Verification items for the finished model (mm, model axes). Face numbers are marked on the shaded views. A direction names the side the tool comes from. Round coordinates to 2 decimals unless told otherwise and drop trailing zeros. Write each loop counter-clockwise with the first axis right and the second up, starting at its lowest first coordinate (ties: lowest second). Pieces come first, ordered by that corner, then holes. Notation, with made-up numbers: M 86,-36 L 122,-36 A30 cw 122,-8 Z; hole C 7.25,44 d2. An arc over 180 degrees is marked long. Write each question's results on one line, items separated by ' | '.
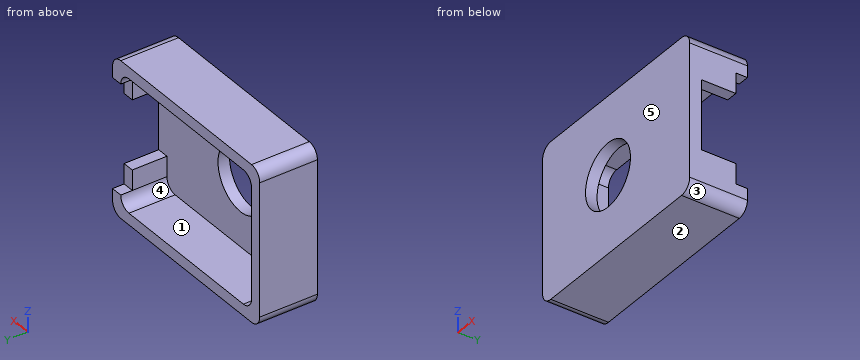
from build123d import *

# Parameters (mm, degrees)
SKETCH1_W           = 36
SKETCH1_H           = 27
SKETCH1_R           = 5.5
BOSS_EXTRUDE1_DEPTH = 2
BOSS_EXTRUDE2_DEPTH = 8
SKETCH3_W           = 3.5
SKETCH3_H           = 6
BOSS_EXTRUDE3_DEPTH = 2
FILLET2_R           = 2


with BuildPart() as part:
    # Sketch1 → Boss-Extrude1 (new body)
    with BuildSketch(Plane(origin=(0, 0, 0), x_dir=(1, 0, 0), z_dir=(0, 1, 0))):
        Rectangle(SKETCH1_W, SKETCH1_H)
        with Locations(Location((-2, 0, 0), (0, 0, 270))):
            Circle(SKETCH1_R, mode=Mode.SUBTRACT)
    extrude(amount=BOSS_EXTRUDE1_DEPTH)

    # Sketch2 → Boss-Extrude2 (add)
    with BuildSketch(Plane(origin=(0, 2, 0), x_dir=(1, 0, 0), z_dir=(0, 1, 0))):
        Polygon((18, 13.5), (-18, 13.5), (-18, -13.5), (18, -13.5), (18, -9.5), (16, -9.5), (16, -11.5), (-16, -11.5), (-16, 11.5), (16, 11.5), (16, 9.5), (18, 9.5), align=None)
    extrude(amount=BOSS_EXTRUDE2_DEPTH)

    # Sketch3 → Boss-Extrude3 (add)
    with BuildSketch(Plane(origin=(18, 0, 0), x_dir=(0, 0, -1), z_dir=(1, 0, 0))):
        with Locations((-7.75, 5)):
            Rectangle(SKETCH3_W, SKETCH3_H)
        with Locations((7.75, 5)):
            Rectangle(SKETCH3_W, SKETCH3_H)
    extrude(amount=-BOSS_EXTRUDE3_DEPTH)

    # Fillet2
    fillet2_edges = [part.edges().sort_by_distance(p)[0] for p in [
        (-18, 5, 13.5),
        (-18, 5, -13.5),
        (18, 5, -13.5),
        (18, 5, 13.5),
        (16, 6, -11.5),
        (16, 6, 11.5),
        (-16, 6, 11.5),
        (-16, 6, -11.5),
    ]]
    fillet(fillet2_edges, radius=FILLET2_R - 0.0001)  # a hair under: the kernel refuses the full size


solid = part.part
1) Sectioned sample at B-B, the plane x = -2. Record the cut outline in (y, z).
Calculated:
outline: M 0,-13.5 L 10,-13.5 L 10,-11.5 L 2,-11.5 L 2,-5.5 L 0,-5.5 Z; M 0,5.5 L 2,5.5 L 2,11.5 L 10,11.5 L 10,13.5 L 0,13.5 Z
2) Draft check along X on the marked faces 1, 2 and 3. Enter one of: pulls with the +X half, pulls with the -X half, needs draft (parallel to the pull), parting line crosses it, or undercut.
Calculated:
face 1: undercut | face 2: needs draft | face 3: pulls with the +X half
3) Sectioned sample at A-A, the plane z = 0. Record the cut outline in (x, y).
Calculated:
outline: M -18,0 L -7.5,0 L -7.5,2 L -16,2 L -16,10 L -18,10 Z; M 3.5,0 L 18,0 L 18,2 L 3.5,2 Z
4) Depth check by flat-ended pin: P1, Ø0.6, axis at x = 16.5, y = 6.5, coming from the -Z side; P2, Ø1, axis at x = 16.5, z = -7.5, coming from the +Y side; P3, Ø3, axis at x = -7.5, z = 9.5, coming from the +Y side. Enter the tip coordinate at first touch or a pass-through.
Calculated:
P1: stops at z = -13.49 | P2: stops at y = 8 | P3: stops at y = 2
5) Sectioned sample at D-D, the plane z = 7. Record the cut outline in (x, y).
Calculated:
outline: M -18,0 L 18,0 L 18,8 L 16,8 L 16,2 L -16,2 L -16,10 L -18,10 Z
6) Access from +Z, -Z, +X, -X, +Y, -Y to the whole of each face (thin tool, end or side, straight path). Record for the marked faces 4 and 5.
Calculated:
face 4: +Y | face 5: +Z, -Z, +X, -X, -Y
7) Material ranges on line 1 (Z direction, x = 6.5, y = 4.25); line 2 (X direction, y = 1.25, z = 0); line 3 (Y direction, x = 0.5, z = 6.25), recorded low to high. Write a range as [from, to].
Calculated:
line 1: z = [-13.5, -11.5], [11.5, 13.5] | line 2: x = [-18, -7.5], [3.5, 18] | line 3: y = [0, 2]
8) Sectioned sample at C-C, the plane y = 1.25. Record the cut outline in (x, z), and give its area (3 significant figures).
Calculated:
outline: M -18,-11.5 A2 ccw -16,-13.5 L 16,-13.5 A2 ccw 18,-11.5 L 18,11.5 A2 ccw 16,13.5 L -16,13.5 A2 ccw -18,11.5 Z; hole C -2,0 d11 | area: 874 mm²
